Source: CAD feature listing. Evaluate the final solid. Frame: model axes, mm. A direction names the side the tool comes from. Give positions to 0.01 mm unless a question says otherwise; leave off trailing zeros. Order: outer loops, then holes, each group sorted by start corner. A loop starts at its lowest first (then second) coordinate and runs counter-clockwise, first axis right, second up. Notation, with made-up numbers: M 43,79 L 89,79 A22 ccw 89,92 Z; hole C 29,9 d2. An arc over 180 degrees is marked long. One line per question, with ' | ' between items. Start each with the question number.
from build123d import *

# Parameters (mm, degrees)
F0_W     = 5
F0_H     = 7
F0_R     = 3
F1_DEPTH = 3


# Not quite as in the source:
# - a feature names something its author has since deleted; it is built from what else it names


with BuildPart() as f1:
    # F0 (on Front) → F1 (new body)
    with BuildSketch(Plane.XZ):
        Polygon((1.3333333333, 0), (0, 0), (0, 7), (-10, 2.5), (-10, -2), (-2, -2), align=None)
        Polygon((0, 7), (0, 0), (1.3333333333, 0), (8, 4), (13, 4), (14.2307692308, 0), (32, 0), (35, 0), (35, 7), align=None)
        Polygon((32, 0), (14.2307692308, 0), (15, -2.5), (11.75, -3.5), (15, -5), align=None)
        with Locations((37.5, 3.5)):
            Rectangle(F0_W, F0_H)
        with BuildLine():
            ThreePointArc((40, 0), (61.4283268073, 3.5), (40, 7))
            Line((40, 7), (40, 0))
        make_face()
        with Locations((57.4283268073, 3.5)):
            Circle(F0_R, mode=Mode.SUBTRACT)
        Polygon((8, 4), (1.3333333333, 0), (14.2307692308, 0), (13, 4), align=None)
        Polygon((14.2307692308, 0), (1.3333333333, 0), (-2, -2), (-10, -2), (-10, 2.5), (0, 7), (35, 7), (35, 8), (-12, 8), (-12, -6), (35, -6), (35, 0), (32, 0), (15, -5), (11.75, -3.5), (15, -2.5), align=None)
        with Locations((57.4283268073, 3.5)):
            Circle(F0_R)
    extrude(amount=F1_DEPTH)


solid = f1.part
Item 1: Reachability of faces 1 (the flat face through (37, -1, 0)), 2 (the flat face through (12, -1, 8)), 3 (the flat face through (11, -1, -6)) from +Z, -Z, +X, -X, +Y, -Y: full face, straight path, thin tool, end or side. Return the list, or none.
Item 2: Cut plane A-A on y = -1.05. Return the cut outline in (x, z).
Item 3: Cut plane B-B on x = 33.5. Return the cut outline in (y, z), and give its area (3 significant figures).
Item 4: Mould query, pull axis X, two halves, no side actions, for faces 4 (the flat face through (24, -3, 1)), 5 (the flat face through (38, -1, 7)), 6 (the flat face through (-12, -1, 1)). Classes: pulls with the +X half, pulls with the -X half, needs draft (parallel to the pull), parting line crosses it, or undercut.
Item 5: Line query: line 1 (Z direction, x = 51, y = -0.2); line 2 (X direction, y = -0.3, z = 3); line 3 (X direction, y = -0.8, z = 7.5). Output: solid intervals per line, ascending.
Item 6: Pin query (flat end, axial travel): pin 1 Ø0.8 at (y, z) = (-2, 7.5) entering from +X; pin 2 Ø6 at (x, z) = (9.5, -0.5) entering from +Y; pin 3 Ø0.9 at (x, y) = (15.5, -1) entering from +Z. Return the tip coordinate at first contact, or that it passes through.
Results are:
1) face 1: -Z, +Y, -Y | face 2: +Z, -X, +Y, -Y | face 3: -Z, -X, +Y, -Y
2) outline: M -12,-6 L 35,-6 L 35,0 L 40,0 A11 ccw long 40,7 L 35,7 L 35,8 L -12,8 Z
3) outline: M -3,-6 L 0,-6 L 0,8 L -3,8 Z | area: 42.0 mm2
4) face 4: needs draft | face 5: undercut | face 6: pulls with the -X half
5) line 1: z = -7.49 to 14.49 | line 2: x = -12 to 61.42 | line 3: x = -12 to 35, 40.18 to 60.68
6) pin 1: stops at x = 60.82 | pin 2: stops at y = 0 | pin 3: stops at z = 8
